Model file for the job. Use its own axes, mm. Coordinates: 2 decimals unless noted, no trailing zeros. Write each loop counter-clockwise with the first axis right and the second up, starting at its lowest first coordinate (ties: lowest second). Pieces come first, ordered by that corner, then holes. Notation, with made-up numbers: (-33.75, 20) - (19.25, 20) arc R18 cw to (19.25, 37) - close; hole circle Ø2 at (12.5, 23). An arc over 180 degrees is marked (long way). Put each result on its own line as item: value. Start each with the question number.
1. Saw through at A-A, the plane y = 0. Write the cut outline in (x, z).
2. Drill centre lines: L1, parallel to Y at x = 267, z = 0; L2, parallel to Z at x = 188, y = 2.25. Where is each one in solid material? Low to high. Write a range as from..to.
3. Drop flat-ended pins along their axis: P1, Ø2, axis at x = 277.5, z = 9, coming from the +Y side; P2, Ø1.5, axis at y = 1, z = -10, coming from the +X side; P3, Ø4, axis at x = 166.5, y = 4.5, coming from the +Z side. Give the stop position or say it passes through.
4. Saw through at C-C, the plane x = 117.5. Write the cut outline in (y, z), plus the area to 3 significant figures.
```python
from build123d import *

# Parameters (mm, degrees)
F0_R     = 12.7
F1_DEPTH = 279.4
F3_DEPTH = 2.54
F4_R     = 6.345743
F5_DEPTH = 25.4


with BuildPart() as f1:
    # F0 (on Right) → F1 (new body)
    with BuildSketch(Plane.YZ):
        Circle(F0_R)
    extrude(amount=F1_DEPTH)

    # F2 (on face) → F3 (cut)
    with BuildSketch(Plane.YZ.offset(279.4)):
        with BuildLine():
            Line((17.428713, 2.54), (12.443408, 2.54))
            ThreePointArc((12.443408, 2.54), (12.635689, 1.276464), (12.7, 0))
            ThreePointArc((12.7, 0), (12.635689, -1.276464), (12.443408, -2.54))
            Line((12.443408, -2.54), (17.428713, -2.54))
            Line((17.428713, -2.54), (17.428713, 2.54))
        make_face()
        with BuildLine():
            ThreePointArc((-2.54, 12.443408), (0, 12.7), (2.54, 12.443408))
            Line((2.54, 12.443408), (2.54, 18.02417))
            Line((2.54, 18.02417), (-2.54, 18.02417))
            Line((-2.54, 18.02417), (-2.54, 12.443408))
        make_face()
        with BuildLine():
            ThreePointArc((-12.443408, -2.54), (-12.7, 0), (-12.443408, 2.54))
            Line((-12.443408, 2.54), (-17.28948, 2.54))
            Line((-17.28948, 2.54), (-17.28948, -2.54))
            Line((-17.28948, -2.54), (-12.443408, -2.54))
        make_face()
        with BuildLine():
            Line((2.54, -17.407856), (2.54, -12.443408))
            ThreePointArc((2.54, -12.443408), (0, -12.7), (-2.54, -12.443408))
            Line((-2.54, -12.443408), (-2.54, -17.407856))
            Line((-2.54, -17.407856), (2.54, -17.407856))
        make_face()
        with BuildLine():
            Line((12.443408, 2.54), (1.335046, 2.54))
            Line((1.335046, 2.54), (1.335046, -2.54))
            Line((1.335046, -2.54), (12.443408, -2.54))
            ThreePointArc((12.443408, -2.54), (12.635689, -1.276464), (12.7, 0))
            ThreePointArc((12.7, 0), (12.635689, 1.276464), (12.443408, 2.54))
        make_face()
        with BuildLine():
            Line((-2.623477, 2.54), (-12.443408, 2.54))
            ThreePointArc((-12.443408, 2.54), (-12.7, 0), (-12.443408, -2.54))
            Line((-12.443408, -2.54), (-2.623477, -2.54))
            Line((-2.623477, -2.54), (-2.623477, 2.54))
        make_face()
        with BuildLine():
            ThreePointArc((-2.54, -12.443408), (0, -12.7), (2.54, -12.443408))
            Line((2.54, -12.443408), (2.54, -3.909942))
            Line((2.54, -3.909942), (-2.54, -3.909942))
            Line((-2.54, -3.909942), (-2.54, -12.443408))
        make_face()
        with BuildLine():
            Line((2.54, 4.331574), (2.54, 12.443408))
            ThreePointArc((2.54, 12.443408), (0, 12.7), (-2.54, 12.443408))
            Line((-2.54, 12.443408), (-2.54, 4.331574))
            Line((-2.54, 4.331574), (2.54, 4.331574))
        make_face()
    extrude(amount=-F3_DEPTH, mode=Mode.SUBTRACT)

    # F4 (on face) → F5 (cut)
    with BuildSketch(Plane.YZ.offset(279.4)):
        Circle(F4_R)
    extrude(amount=-F5_DEPTH, mode=Mode.SUBTRACT)


solid = f1.part
```
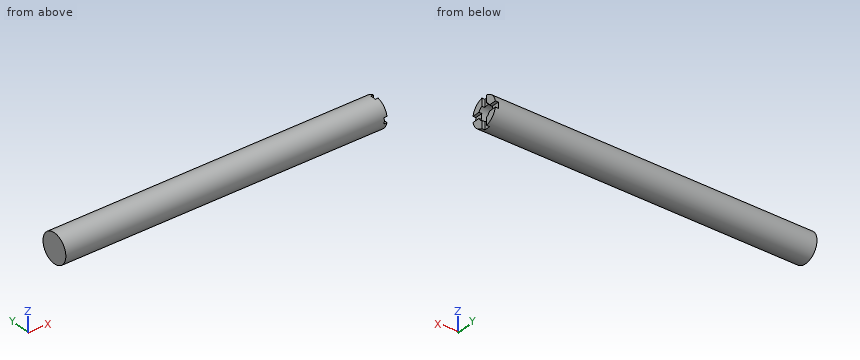
Final values:
1. outline: (0, -12.7) - (276.86, -12.7) - (276.86, -6.35) - (254, -6.35) - (254, 6.35) - (276.86, 6.35) - (276.86, 12.7) - (0, 12.7) - close
2. L1: y = -12.7..-6.35, 6.35..12.7
2. L2: z = -12.5..12.5
3. P1: stops at y = 9.86
3. P2: stops at x = 276.86
3. P3: stops at z = 12.45
4. outline: circle Ø25.4 at (0, 0)
4. area: 507 mm²
